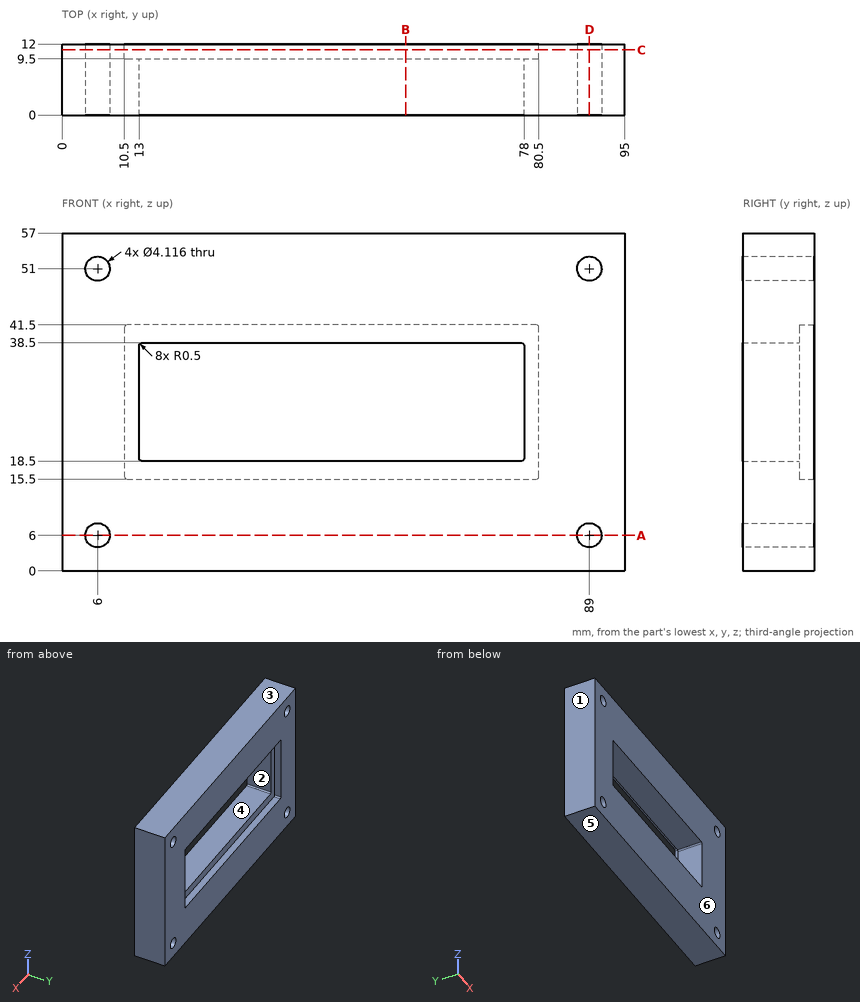
Drawing for the job (mm, zero at the part's lowest x, y, z). A direction names the side the tool comes from. Round coordinates to 2 decimals unless told otherwise and drop trailing zeros. Loops run counter-clockwise (first coordinate to the right, second up) from the corner with the lowest first, then second, coordinate; pieces in that order, holes last. Notation, with made-up numbers: (22.25, 49) -> (26.25, 49) arc R18 cw to (26.25, 79) -> close; hole circle Ø3 at (35.25, 50). An arc over 180 degrees is marked (long way). Use one line per item in the form item = value. Start each with the question number.
Item 1: Two-plate mould, pull along Z, no slides. Class the marked faces 3, 4, 5 and 6: released by +Z, released by -Z, zero draft, split by the parting line, or undercut.
Item 2: Drill centre lines: line 1 along X through (y, z) = (8.5, 51); line 2 along Z through (x, y) = (89, 3); line 3 along Z through (x, y) = (75, 11.25). Where is each one in solid material? Low to high.
Item 3: Tool access for the marked faces 1 and 2: list every direction of +Z, -Z, +X, -X, +Y, -Y with a clear straight run to the whole face (end or side of a thin tool).
Item 4: Drop a flat-ended pin along its axis: pin 1 Ø1.5 at (x, y) = (85, 10.5) entering from -Z. Give the stop position or say it passes through.
Item 5: Band-saw the part on B-B (x = 58). List the corners of the cut face in (y, z).
Item 6: Band-saw the part on A-A (z = 6). List the corners of the cut face in (x, y).
Item 7: Band-saw the part on C-C (y = 11). List the corners of the cut face in (x, z).
Item 8: Band-saw the part on D-D (x = 89). List the corners of the cut face in (y, z), plus the area to 3 significant figures.
Data:
q1.face_3 = released by +Z
q1.face_4 = undercut
q1.face_5 = released by -Z
q1.face_6 = zero draft
q2.line_1 = 0 to 3.94, 8.06 to 86.94, 91.06 to 95
q2.line_2 = 0 to 3.94, 8.06 to 48.94, 53.06 to 57
q2.line_3 = 0 to 15.5, 41.5 to 57
q3.face_1 = +Z, -Z, -X, +Y, -Y
q3.face_2 = +Y, -Y
q4.pin_1 = 0
q5.outline = (0, 0) -> (12, 0) -> (12, 15.5) -> (9.5, 15.5) -> (9.5, 18.5) -> (0, 18.5) -> close; (0, 38.5) -> (9.5, 38.5) -> (9.5, 41.5) -> (12, 41.5) -> (12, 57) -> (0, 57) -> close
q6.outline = (0, 0) -> (3.94, 0) -> (3.94, 12) -> (0, 12) -> close; (8.06, 0) -> (86.94, 0) -> (86.94, 12) -> (8.06, 12) -> close; (91.06, 0) -> (95, 0) -> (95, 12) -> (91.06, 12) -> close
q7.outline = (0, 0) -> (95, 0) -> (95, 57) -> (0, 57) -> close; hole circle Ø4.12 at (6, 6); hole circle Ø4.12 at (6, 51); hole (10.5, 16) arc R0.5 ccw to (11, 15.5) -> (80, 15.5) arc R0.5 ccw to (80.5, 16) -> (80.5, 41) arc R0.5 ccw to (80, 41.5) -> (11, 41.5) arc R0.5 ccw to (10.5, 41) -> close; hole circle Ø4.12 at (89, 6); hole circle Ø4.12 at (89, 51)
q8.outline = (0, 0) -> (12, 0) -> (12, 3.94) -> (0, 3.94) -> close; (0, 8.06) -> (12, 8.06) -> (12, 48.94) -> (0, 48.94) -> close; (0, 53.06) -> (12, 53.06) -> (12, 57) -> (0, 57) -> close
q8.area = 585 mm^2
